Geometry check sheet. Reference: the model listing, model coordinates, mm. A direction names the side the tool comes from. Give positions to 0.01 mm unless a question says otherwise; leave off trailing zeros. Order: outer loops, then holes, each group sorted by start corner. A loop starts at its lowest first (then second) coordinate and runs counter-clockwise, first axis right, second up. Notation, with made-up numbers: (82.5, 40) - (111.5, 40) arc R25 cw to (111.5, 60) - close; hole circle Ø4 at (39, 14). An arc over 180 degrees is marked (long way). Put each result on its own line as item: value. Start each with the question number.
Autodesk Inventor part; units mm, degrees
ref_plane "YZ Plane" through (0, 0, 0) normal (1, 0, 0) x (0, 1, 0)
ref_plane "XZ Plane" through (0, 0, 0) normal (0, 1, 0) x (-1, 0, 0)
ref_plane "XY Plane" through (0, 0, 0) normal (0, 0, 1) x (1, 0, 0)
sketch "Sketch1" plane through (0, 0, 0) normal (0, 0, 1) x (1, 0, 0)
  line L0 (0, 0) -> (150, 0)
  line L1 (150, 0) -> (150, 150)
  line L2 (150, 150) -> (0, 150)
  line L3 (0, 150) -> (0, 0)
  dimension "d0" = 150
  dimension "d1" = 150
extrude "Extrusion1" add sketch "Sketch1" along normal blind 8
sketch "Sketch2" plane through (0, 0, 8) normal (0, 0, 1) x (1, 0, 0)
  circle A0 centre (110, 40) radius 24
  line L0 (0, 0) -> (150, 0)
  line L1 (150, 0) -> (150, 150)
  line L2 (110, 40) -> (55, 40)
  circle A1 centre (55, 40) radius 2
  dimension "d4" = 48
  dimension "d5" = 40
  dimension "d6" = 40
  dimension "d7" = 55
  dimension "d8" = 4
extrude "Extrusion2" cut sketch "Sketch2" against normal blind 8
sketch "Sketch3" plane through (0, 0, 8) normal (0, 0, 1) x (1, 0, 0)
  circle A0 centre (110, 40) radius 26
  point P0 (0, 0)
  dimension "d12" = 52
extrude "Extrusion3" cut sketch "Sketch3" against normal blind 7
properties part number "cote droit"
Item 1: Cross-section at C-C (z = 3). Enter the section's corners in (x, y).
Item 2: Release check for a two-part mould opening along X. For faces 1 (the face through (55, 38, 4)), 2 (the face through (0, 76, 4)), 3 (the face through (74, 76, 8)) record: +X half, -X half, draft (parallel to the pull), parting line (faces both ways), or undercut.
Item 3: Set-up check for faces 4 (the face through (84.025, 41.143, 4.549)), 5 (the face through (90.95, 25.4, 0.51)): record each of +Z, -Z, +X, -X, +Y, -Y from which the full face is reachable in a straight line by a thin tool's end or side.
Item 4: Thickness scan on line 1 along X through (y, z) = (50, 6.5); line 2 along Y through (x, z) = (110, 3.5); line 3 along Y through (x, z) = (110, 0.35). Record the ranges inside material, lowest first.
Item 5: Cross-section at B-B (y = 40). Enter the section's corners in (x, z).
Item 6: Cross-section at D-D (x = 55). Enter the section's corners in (y, z).
Item 7: Cross-section at A-A (x = 110). Enter the section's corners in (y, z), and give its area (3 significant figures).
Recorded:
1. outline: (0, 0) - (150, 0) - (150, 150) - (0, 150) - close; hole circle Ø4 at (55, 40); hole circle Ø52 at (110, 40)
2. face 1: undercut
2. face 2: -X half
2. face 3: draft
3. face 4: +Z
3. face 5: +Z, -Z
4. line 1: x = 0 to 86, 134 to 150
4. line 2: y = 0 to 14, 66 to 150
4. line 3: y = 0 to 16, 64 to 150
5. outline: (0, 0) - (53, 0) - (53, 8) - (0, 8) - close; (57, 0) - (86, 0) - (86, 1) - (84, 1) - (84, 8) - (57, 8) - close; (134, 0) - (150, 0) - (150, 8) - (136, 8) - (136, 1) - (134, 1) - close
6. outline: (0, 0) - (38, 0) - (38, 8) - (0, 8) - close; (42, 0) - (150, 0) - (150, 8) - (42, 8) - close
7. outline: (0, 0) - (16, 0) - (16, 1) - (14, 1) - (14, 8) - (0, 8) - close; (64, 0) - (150, 0) - (150, 8) - (66, 8) - (66, 1) - (64, 1) - close
7. area: 788 mm^2
